Read the model definition and answer for the solid it produces. Units are mm, in the model's axes. Give positions to 0.01 mm unless a question says otherwise; leave off trailing zeros. Order: outer loops, then holes, each group sorted by start corner. A loop starts at its lowest first (then second) coordinate and runs counter-clockwise, first axis right, second up. Notation, with made-up numbers: (54, 59) - (109, 59) arc R24 cw to (109, 80) - close; hole circle Ø6 at (62, -21.75). An arc over 180 degrees is marked (long way). Write each question's results on one line, items separated by ' | '. Start each with the question number.
Q1. For a pull along Z with two mould halves and no side action, classify faces 1 (the face through (-17.3, 1.6, 63.4)), 2 (the face through (-21, 2, 50.455)), 3 (the face through (-32.6, 1.6, 5.2)) as +Z half, -Z half, draft (parallel to the pull), parting line (faces both ways), or undercut.
Q2. Find section C-C on z = 0.5. Give the vertices of the cut face in (x, y) (3 decimals).
Q3. Find the intervals of material crossed by line 1 along Z through (x, y) = (6.5, 0.4); line 2 along Z through (x, y) = (-18, 1.05); line 3 along Z through (x, y) = (20, 1.6), in increasing order. Write a range as from..to.
Q4. Find section B-B on x = -34. Give the vertices of the cut face in (y, z) (3 decimals).
Q5. Find section A-A on z = 12. Give the vertices of the cut face in (x, y) (3 decimals), and give its area (3 significant figures).
Q6. Find section D-D on y = 2.5. Count the separate pieces of the cut face and the enclosed holes in it, and give its area (3 significant figures).
Q7. A flat-ended cylindrical pin translates along its axis: P1, Ø5, axis at x = 6.75, z = 56.95, coming from the +Y side (3 decimals). Find the tip coordinate at first contact, or state that the pin passes through.
from build123d import *

# Parameters (mm, degrees)
SKETCH1_R           = 1.5
SKETCH1_R_2         = 2
SKETCH1_W           = 2.5
SKETCH1_H           = 14.5
SKETCH1_W_2         = 14.5
SKETCH1_H_2         = 2.5
SKETCH1_W_3         = 17.8
SKETCH1_H_3         = 43.18
BOSS_EXTRUDE1_DEPTH = 3.175


with BuildPart() as part:
    # Sketch1 → Boss-Extrude1 (new body)
    with BuildSketch(Plane(origin=(0, 0, 0), x_dir=(1, 0, 0), z_dir=(0, 1, 0))):
        Polygon((-22.047586286, 28.724844999), (28.152410312, 28.724844999), (28.152410312, -68.278843574), (-6.847589688, -68.278843574), (-28.119391264, -58.34898159), (-42.847468938, -38.147899243), align=None)
        with Locations((25.652410312, 26.224844999)):
            Circle(SKETCH1_R, mode=Mode.SUBTRACT)
        with Locations((25.652410312, -65.778843574)):
            Circle(SKETCH1_R, mode=Mode.SUBTRACT)
        with Locations((-38.087063045, -37.694179546)):
            Circle(SKETCH1_R, mode=Mode.SUBTRACT)
        with Locations((-18.207043121, 26.221156426)):
            Circle(SKETCH1_R, mode=Mode.SUBTRACT)
        with Locations((-24.448175277, -56.401325246)):
            Circle(SKETCH1_R, mode=Mode.SUBTRACT)
        with Locations((16.902410312, 21.724844999)):
            Circle(SKETCH1_R_2, mode=Mode.SUBTRACT)
        with Locations((11.902410312, 21.724844999)):
            Circle(SKETCH1_R_2, mode=Mode.SUBTRACT)
        with Locations((4.202410312, 21.724844999)):
            Circle(SKETCH1_R_2, mode=Mode.SUBTRACT)
        with Locations((-0.797589688, 21.724844999)):
            Circle(SKETCH1_R_2, mode=Mode.SUBTRACT)
        with Locations((-8.518099948, 19.221156426)):
            Circle(SKETCH1_R_2, mode=Mode.SUBTRACT)
        with Locations((-13.518099948, 19.221156426)):
            Circle(SKETCH1_R_2, mode=Mode.SUBTRACT)
        with Locations((-16.301455712, 9.146912193)):
            Circle(SKETCH1_R_2, mode=Mode.SUBTRACT)
        with Locations((-21.301455712, 9.146912193)):
            Circle(SKETCH1_R_2, mode=Mode.SUBTRACT)
        with Locations((-2.047589688, -61.948843574)):
            Circle(SKETCH1_R_2, mode=Mode.SUBTRACT)
        with Locations((-2.047589688, -56.948843574)):
            Circle(SKETCH1_R_2, mode=Mode.SUBTRACT)
        with Locations((6.752410312, -61.948843574)):
            Circle(SKETCH1_R_2, mode=Mode.SUBTRACT)
        with Locations((6.752410312, -56.948843574)):
            Circle(SKETCH1_R_2, mode=Mode.SUBTRACT)
        with Locations((-8.847589688, -59.278843574)):
            Circle(SKETCH1_R_2, mode=Mode.SUBTRACT)
        with Locations((-13.847589688, -59.278843574)):
            Circle(SKETCH1_R_2, mode=Mode.SUBTRACT)
        with Locations((21.452410312, 8.724844999)):
            Circle(SKETCH1_R_2, mode=Mode.SUBTRACT)
        with Locations((16.452410312, 8.724844999)):
            Circle(SKETCH1_R_2, mode=Mode.SUBTRACT)
        with Locations((6.352410312, 8.724844999)):
            Circle(SKETCH1_R_2, mode=Mode.SUBTRACT)
        with Locations((1.352410312, 8.724844999)):
            Circle(SKETCH1_R_2, mode=Mode.SUBTRACT)
        with Locations((14.352410312, -4.275155001)):
            Circle(SKETCH1_R_2, mode=Mode.SUBTRACT)
        with Locations((19.352410312, -4.275155001)):
            Circle(SKETCH1_R_2, mode=Mode.SUBTRACT)
        with Locations((3.352410312, -4.275155001)):
            Circle(SKETCH1_R_2, mode=Mode.SUBTRACT)
        with Locations((-1.647589688, -4.275155001)):
            Circle(SKETCH1_R_2, mode=Mode.SUBTRACT)
        with Locations((16.652410312, -23.778843574)):
            Circle(SKETCH1_R_2, mode=Mode.SUBTRACT)
        with Locations((11.652410312, -23.778843574)):
            Circle(SKETCH1_R_2, mode=Mode.SUBTRACT)
        with Locations((0.902410312, -23.778843574)):
            Circle(SKETCH1_R_2, mode=Mode.SUBTRACT)
        with Locations((-4.097589688, -23.778843574)):
            Circle(SKETCH1_R_2, mode=Mode.SUBTRACT)
        with Locations((19.452410312, -40.334046802)):
            Circle(SKETCH1_R_2, mode=Mode.SUBTRACT)
        with Locations((14.452410312, -40.334046802)):
            Circle(SKETCH1_R_2, mode=Mode.SUBTRACT)
        with Locations((1.752410312, -40.334046802)):
            Circle(SKETCH1_R_2, mode=Mode.SUBTRACT)
        with Locations((-3.247589688, -40.334046802)):
            Circle(SKETCH1_R_2, mode=Mode.SUBTRACT)
        with Locations((16.902410312, -59.278843574)):
            Circle(SKETCH1_R_2, mode=Mode.SUBTRACT)
        with Locations((16.902410312, -64.278843574)):
            Circle(SKETCH1_R_2, mode=Mode.SUBTRACT)
        with Locations((-8.497589688, -30.725155001)):
            Rectangle(SKETCH1_W, SKETCH1_H, mode=Mode.SUBTRACT)
        with Locations((3.342410312, -31.528843574)):
            Rectangle(SKETCH1_W_2, SKETCH1_H_2, mode=Mode.SUBTRACT)
        with Locations((-21.247589688, -28.865155001)):
            Rectangle(SKETCH1_W_3, SKETCH1_H_3, mode=Mode.SUBTRACT)
    extrude(amount=BOSS_EXTRUDE1_DEPTH)


solid = part.part
Working result:
1) face 1: +Z half | face 2: undercut | face 3: -Z half
2) outline: (-31.138, 0) - (28.152, 0) - (28.152, 3.175) - (-31.138, 3.175) - close
3) line 1: -28.72..-10.72, -6.73..30.28, 32.78..54.96, 58.93..59.96, 63.93..68.28 | line 2: -28.72..-27.71, -24.74..-10.2, -8.09..7.28, 50.46..63.07 | line 3: -28.72..-10.1, -7.35..2.38, 6.17..38.41, 42.26..68.28
4) outline: (0, 9.703) - (3.175, 9.703) - (3.175, 50.283) - (0, 50.283) - close
5) outline: (-34.715, 0) - (-30.148, 0) - (-30.148, 3.175) - (-34.715, 3.175) - close; (-12.348, 0) - (28.152, 0) - (28.152, 3.175) - (-12.348, 3.175) - close | area: 143 mm²
6) separate pieces: 1 | enclosed holes: 40 | area: 4,510 mm²
7) P1: y = 3.175
